Part model, mm, in its own coordinate system. Face numbers are marked on the shaded views. A direction names the side the tool comes from. Coordinates: 2 decimals unless noted, no trailing zeros. Loops run counter-clockwise (first coordinate to the right, second up) from the corner with the lowest first, then second, coordinate; pieces in that order, holes last. Notation, with made-up numbers: (54, -18) - (83, -18) arc R33 ccw to (83, 16) - close; hole circle Ø10 at (-33.5, 50). An arc over 180 degrees is marked (long way). Use a Markdown table: item, result. Add a question column.
1) Band-saw the part on A-A (z = 24.5). Give the cut face in (x, y).
2) Pull direction Y, two halves, no side cores. Call the marked faces 1, 2 and 3: +Y half, -Y half, draft (parallel to the pull), parting line (faces both ways), or undercut.
3) Band-saw the part on B-B (x = 1). Give the cut face in (y, z), plus the area to 3 significant figures.
4) Tool access for the marked faces 4 and 5: list every direction of +Z, -Z, +X, -X, +Y, -Y with a clear straight run to the whole face (end or side of a thin tool).
5) Band-saw the part on C-C (x = 45.5). Give the cut face in (y, z), plus the area to 3 significant figures.
6) Drop flat-ended pins along their axis: P1, Ø1.2, axis at y = 19, z = 19.5, coming from the -X side; P2, Ø5, axis at x = 21.17, z = 29.92, coming from the -Y side; P3, Ø1.6, axis at x = 9, y = 19.5, coming from the +Z side; P4, Ø3, axis at x = 39, y = 17, coming from the +Z side. Give the stop position or say it passes through.
7) Probe probe 1 along X at (y, z) = (19, 31); probe 2 along X at (y, z) = (6.5, 42); probe 3 along Y at (x, z) = (11, 11.5). List the from-to ranges inside material, lowest first. Write a range as [from, to].
8) Band-saw the part on D-D (z = 8.5). Give the cut face in (x, y), plus the area to 3 significant figures.
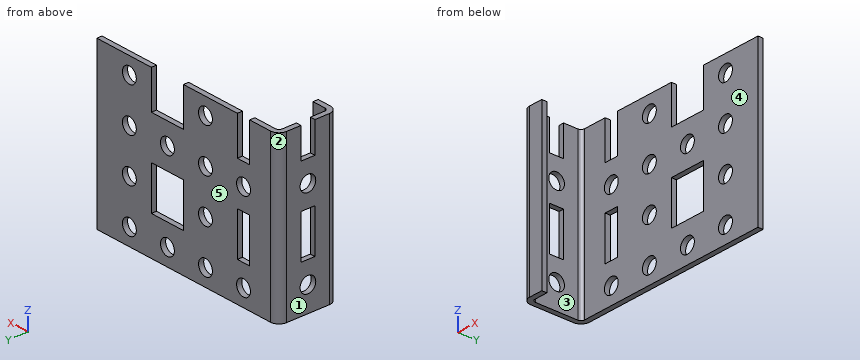
from build123d import *

# Parameters (mm, degrees)
F0_W     = 1.5
F0_H     = 1.5
F0_W_2   = 58
F0_H_2   = 14.4
F0_W_3   = 4.95
F1_DEPTH = 47.24
F2_R     = 2.5
F3_R     = 1
F4_R     = 2.275
F4_W     = 10.55
F4_H     = 12.55
F4_W_2   = 4.05
F5_DEPTH = 17.401
F6_W     = 4.05
F6_H     = 8.825
F6_R     = 2.275
F6_H_2   = 12.55
F7_DEPTH = 25


with BuildPart() as f1:
    # F0 (on Top) → F1 (new body)
    with BuildSketch(Plane.XY):
        with Locations((-1.908001, 19.432347)):
            Rectangle(F0_W, F0_H)
        with Locations((27.841999, 19.432347)):
            Rectangle(F0_W_2, F0_H)
        with Locations((-1.908001, 11.482347)):
            Rectangle(F0_W, F0_H_2)
        with Locations((-1.908001, 3.532347)):
            Rectangle(F0_W, F0_H)
        with Locations((1.316999, 3.532347)):
            Rectangle(F0_W_3, F0_H)
    extrude(amount=F1_DEPTH)

    # F2
    f2_edges = [f1.edges().sort_by_distance(p)[0] for p in [
        (-2.658001, 20.182347, 23.62),
        (-2.658001, 2.782347, 23.62),
    ]]
    fillet(f2_edges, radius=F2_R)

    # F3
    f3_edges = [f1.edges().sort_by_distance(p)[0] for p in [
        (-1.158001, 4.282347, 23.62),
        (-1.158001, 18.682347, 23.62),
    ]]
    fillet(f3_edges, radius=F3_R)

    # F4 (on face) → F5 (cut, through all)
    with BuildSketch(Plane(origin=(0, 20.182347, 0), x_dir=(-1, 0, 0), z_dir=(0, 1, 0))):
        with Locations((-46.166999, 42.415)):
            Circle(F4_R)
        with Locations((-21.166999, 42.415)):
            Circle(F4_R)
        with Locations((-21.166999, 29.915)):
            Circle(F4_R)
        with Locations((-46.166999, 29.915)):
            Circle(F4_R)
        with Locations((-21.166999, 17.415)):
            Circle(F4_R)
        with Locations((-46.166999, 17.415)):
            Circle(F4_R)
        with Locations((-21.166999, 4.915)):
            Circle(F4_R)
        with Locations((-46.166999, 4.915)):
            Circle(F4_R)
        with Locations((-33.666999, 29.915)):
            Circle(F4_R)
        with Locations((-33.666999, 4.915)):
            Circle(F4_R)
        with Locations((-8.666999, 29.915)):
            Circle(F4_R)
        with Locations((-8.666999, 4.915)):
            Circle(F4_R)
        with Locations((-33.666999, 17.415)):
            Rectangle(F4_W, F4_H)
        with Locations((-33.666999, 42.415)):
            Rectangle(F4_W, F4_H)
        with Locations((-8.666999, 17.415)):
            Rectangle(F4_W_2, F4_H)
        with Locations((-8.666999, 42.415)):
            Rectangle(F4_W_2, F4_H)
    extrude(amount=-F5_DEPTH, mode=Mode.SUBTRACT)

    # F6 (on face) → F7 (cut)
    with BuildSketch(Plane(origin=(-2.658001, 0, 0), x_dir=(0, -1, 0), z_dir=(-1, 0, 0))):
        with Locations((-11.482347, 42.8275)):
            Rectangle(F6_W, F6_H)
        with Locations((-11.482347, 32.19)):
            Circle(F6_R)
        with Locations((-11.482347, 19.69)):
            Rectangle(F6_W, F6_H_2)
        with Locations((-11.482347, 7.19)):
            Circle(F6_R)
    extrude(amount=-F7_DEPTH, mode=Mode.SUBTRACT)


solid = f1.part
Answer block:
| question | item | result |
|---|---|---|
| 1 | outline | (-2.66, 5.28) arc R2.5 ccw to (-0.16, 2.78) - (3.79, 2.78) - (3.79, 4.28) - (-0.16, 4.28) arc R1 cw to (-1.16, 5.28) - (-1.16, 9.46) - (-2.66, 9.46) - close; (-2.66, 13.51) - (-1.16, 13.51) - (-1.16, 17.68) arc R1 cw to (-0.16, 18.68) - (56.84, 18.68) - (56.84, 20.18) - (-0.16, 20.18) arc R2.5 ccw to (-2.66, 17.68) - close |
| 2 | face 1 | draft |
| 2 | face 2 | +Y half |
| 2 | face 3 | undercut |
| 3 | outline | (2.78, 0) - (4.28, 0) - (4.28, 47.24) - (2.78, 47.24) - close; (18.68, 0) - (20.18, 0) - (20.18, 47.24) - (18.68, 47.24) - close |
| 3 | area | 142 mm2 |
| 4 | face 4 | +Z, -Z, +X |
| 4 | face 5 | +Z, -Z, +X, -X, +Y |
| 5 | outline | (18.68, 0) - (20.18, 0) - (20.18, 2.74) - (18.68, 2.74) - close; (18.68, 7.09) - (20.18, 7.09) - (20.18, 15.24) - (18.68, 15.24) - close; (18.68, 19.59) - (20.18, 19.59) - (20.18, 27.74) - (18.68, 27.74) - close; (18.68, 32.09) - (20.18, 32.09) - (20.18, 40.24) - (18.68, 40.24) - close; (18.68, 44.59) - (20.18, 44.59) - (20.18, 47.24) - (18.68, 47.24) - close |
| 5 | area | 44.8 mm2 |
| 6 | P1 | x = -2.55 |
| 6 | P2 | y = 18.68 |
| 6 | P3 | z = 36.14 |
| 6 | P4 | through |
| 7 | probe 1 | [-2.28, 6.67], [10.67, 19.17], [23.17, 31.67], [35.67, 44.17], [48.17, 56.84] |
| 7 | probe 2 | [-2.66, -1.16] |
| 7 | probe 3 | [18.68, 20.18] |
| 8 | outline | (-2.66, 5.28) arc R2.5 ccw to (-0.16, 2.78) - (3.79, 2.78) - (3.79, 4.28) - (-0.16, 4.28) arc R1 cw to (-1.16, 5.28) - (-1.16, 9.62) - (-2.66, 9.62) - close; (-2.66, 13.34) - (-1.16, 13.34) - (-1.16, 17.68) arc R1 cw to (-0.16, 18.68) - (56.84, 18.68) - (56.84, 20.18) - (-0.16, 20.18) arc R2.5 ccw to (-2.66, 17.68) - close |
| 8 | area | 113 mm2 |
